Input: part model. Units: mm. Frame: model coordinates. Face numbers are marked on the shaded views. A direction names the side the tool comes from. Give positions to 0.01 mm unless a question says otherwise; leave off trailing zeros. Write each loop counter-clockwise with the first axis right and the second up, starting at its lowest first coordinate (ties: lowest second). Pieces come first, ordered by that corner, then holes. Notation, with made-up numbers: (-22.75, 47.25) - (-5.75, 47.25) arc R16 ccw to (-5.75, 53.25) - close; hole circle Ø2 at (6, 36.25). An arc over 180 degrees is marked (long way). Use a Markdown table: item, result. Add a question column.
1. Section query C-C, the plane z = -0.65. Return loops of the section in (x, y).
2. Set-up query: the marked faces 1, 2, 3, 4 and 5. Return all of +Z, -Z, +X, -X, +Y, -Y with unobstructed straight access to the full face (end or side cutting, diameter ignored); none if empty.
3. Section query A-A, the plane y = 1.5. Return loops of the section in (x, z), plus the area to 3 significant figures.
4. Section query D-D, the plane z = 2. Return loops of the section in (x, y).
5. Section query B-B, the plane x = 1.8. Return loops of the section in (y, z).
6. Pin query (flat end, axial travel): pin 1 (0.5 mm diameter, centred on x = -1.5, z = 2, fed in from +Y); pin 2 (1 mm diameter, centred on x = -1.5, y = 0, fed in from +Z). Return the tip coordinate at first contact, or that it passes through.
7. Material intervals for probe 1 along Y at (x, z) = (-1.65, 0.65); probe 2 along X at (y, z) = (-0.75, -1.9), sorted ascending.
8. Mould query, pull axis Y, two halves, no side actions, for the marked faces 6, 7 and 8. Classes: released by +Y, released by -Y, zero draft, split by the parting line, or undercut.
```python
from build123d import *

# Parameters (mm, degrees)
SKETCH1_W           = 6
SKETCH1_H           = 6
SKETCH1_W_2         = 4.2
SKETCH1_H_2         = 4.2
BOSS_EXTRUDE1_DEPTH = 2.5
SKETCH2_W           = 6
SKETCH2_H           = 10
BOSS_EXTRUDE2_DEPTH = 1.5


with BuildPart() as part:
    # Sketch1 → Boss-Extrude1 (new, symmetric)
    with BuildSketch(Plane.XY):
        Rectangle(SKETCH1_W, SKETCH1_H)
        Rectangle(SKETCH1_W_2, SKETCH1_H_2, mode=Mode.SUBTRACT)
    extrude(amount=BOSS_EXTRUDE1_DEPTH, both=True)

    # Sketch2 → Boss-Extrude2 (add, symmetric)
    with BuildSketch(Plane.XY):
        with Locations((0, 8)):
            Rectangle(SKETCH2_W, SKETCH2_H)
    extrude(amount=BOSS_EXTRUDE2_DEPTH, both=True)


solid = part.part
```
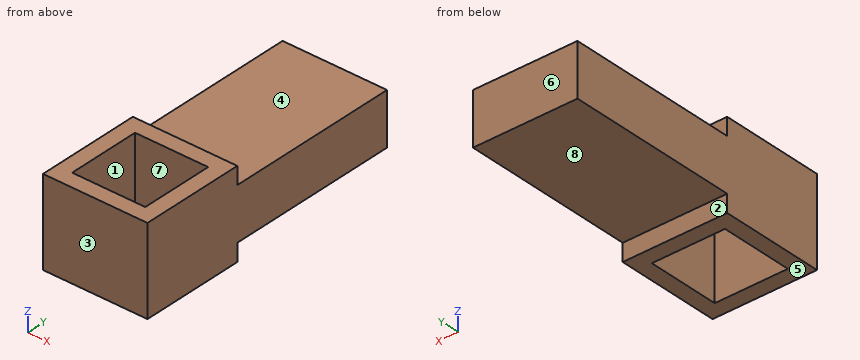
Result sheet:
| question | item | result |
|---|---|---|
| 1 | outline | (-3, -3) - (3, -3) - (3, 13) - (-3, 13) - close; hole (-2.1, -2.1) - (2.1, -2.1) - (2.1, 2.1) - (-2.1, 2.1) - close |
| 2 | face 1 | +Z, -Z |
| 2 | face 2 | -Z, +X, -X, +Y |
| 2 | face 3 | +Z, -Z, +X, -X, -Y |
| 2 | face 4 | +Z, +X, -X, +Y |
| 2 | face 5 | -Z, +X, -X, +Y, -Y |
| 3 | outline | (-3, -2.5) - (-2.1, -2.5) - (-2.1, 2.5) - (-3, 2.5) - close; (2.1, -2.5) - (3, -2.5) - (3, 2.5) - (2.1, 2.5) - close |
| 3 | area | 9.00 mm² |
| 4 | outline | (-3, -3) - (3, -3) - (3, 3) - (-3, 3) - close; hole (-2.1, -2.1) - (2.1, -2.1) - (2.1, 2.1) - (-2.1, 2.1) - close |
| 5 | outline | (-3, -2.5) - (-2.1, -2.5) - (-2.1, 2.5) - (-3, 2.5) - close; (2.1, -2.5) - (3, -2.5) - (3, -1.5) - (13, -1.5) - (13, 1.5) - (3, 1.5) - (3, 2.5) - (2.1, 2.5) - close |
| 6 | pin 1 | stops at y = 3 |
| 6 | pin 2 | passes through |
| 7 | probe 1 | y = -3 to -2.1, 2.1 to 13 |
| 7 | probe 2 | x = -3 to -2.1, 2.1 to 3 |
| 8 | face 6 | released by +Y |
| 8 | face 7 | undercut |
| 8 | face 8 | zero draft |
